from build123d import *

# Parameters (mm, degrees)
SKETCH_1_R          = 14.975
EXTRUDE_1_DEPTH     = 7
SKETCH_2_R          = 2.1
CUT_EXTRUDE_1_DEPTH = 10
SKETCH_3_R          = 1.65
CUT_EXTRUDE_2_DEPTH = 10
SKETCH_5_R          = 3.65
CUT_EXTRUDE_3_DEPTH = 4


with BuildPart() as part:
    # 草图1 → 凸台-拉伸1 (new body)
    with BuildSketch(Plane(origin=(0, 0, 0), x_dir=(1, 0, 0), z_dir=(0, 1, 0))):
        with Locations(Location((0, 0, 0), (0, 0, 270))):
            Circle(SKETCH_1_R)
    extrude(amount=EXTRUDE_1_DEPTH)

    # 草图2 → 切除-拉伸1 (cut)
    with BuildSketch(Plane(origin=(0, 7, 0), x_dir=(1, 0, 0), z_dir=(0, 1, 0))):
        with Locations(Location((-5, 0, 0), (0, 0, 270))):
            Circle(SKETCH_2_R)
        with Locations(Location((2.5, 4.330127019, 0), (0, 0, 270))):
            Circle(SKETCH_2_R)
        with Locations(Location((2.5, -4.330127019, 0), (0, 0, 270))):
            Circle(SKETCH_2_R)
    extrude(amount=-CUT_EXTRUDE_1_DEPTH, mode=Mode.SUBTRACT)

    # 草图3 → 切除-拉伸2 (cut)
    with BuildSketch(Plane(origin=(0, 7, 0), x_dir=(1, 0, 0), z_dir=(0, 1, 0))):
        with Locations(Location((0, 11, 0), (0, 0, 270))):
            Circle(SKETCH_3_R)
        with Locations(Location((9.526279442, 5.5, 0), (0, 0, 270))):
            Circle(SKETCH_3_R)
        with Locations(Location((9.526279442, -5.5, 0), (0, 0, 270))):
            Circle(SKETCH_3_R)
        with Locations(Location((0, -11, 0), (0, 0, 270))):
            Circle(SKETCH_3_R)
        with Locations(Location((-9.526279442, -5.5, 0), (0, 0, 270))):
            Circle(SKETCH_3_R)
        with Locations(Location((-9.526279442, 5.5, 0), (0, 0, 270))):
            Circle(SKETCH_3_R)
    extrude(amount=-CUT_EXTRUDE_2_DEPTH, mode=Mode.SUBTRACT)

    # 草图5 → 切除-拉伸3 (cut)
    with BuildSketch(Plane(origin=(0, 7, 0), x_dir=(1, 0, 0), z_dir=(0, 1, 0))):
        with Locations(Location((-5, 0, 0), (0, 0, 270))):
            Circle(SKETCH_5_R)
        with Locations(Location((2.5, 4.330127019, 0), (0, 0, 270))):
            Circle(SKETCH_5_R)
        with Locations(Location((2.5, -4.330127019, 0), (0, 0, 270))):
            Circle(SKETCH_5_R)
    extrude(amount=-CUT_EXTRUDE_3_DEPTH, mode=Mode.SUBTRACT)


solid = part.part
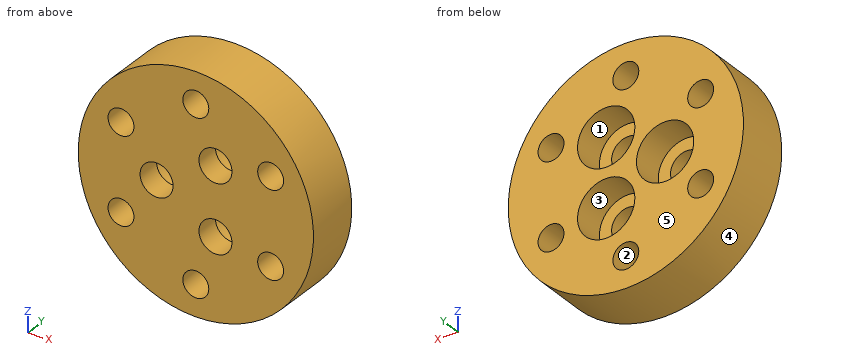
Verification items for the finished model (mm, model axes). Face numbers are marked on the shaded views. A direction names the side the tool comes from. Give positions to 0.01 mm unless a question says otherwise; leave off trailing zeros. Loops run counter-clockwise (first coordinate to the right, second up) from the corner with the lowest first, then second, coordinate; pieces in that order, holes last.
1) Thickness scan on line 1 along X through (y, z) = (2.25, 5.5); line 2 along Z through (x, y) = (4, 1.5); line 3 along X through (y, z) = (4.75, -6.5). Record the ranges inside material, lowest first.
2) Depth check by flat-ended pin: pin 1 Ø1.5 at (y, z) = (4.5, 7) entering from +X; pin 2 Ø2 at (x, z) = (4.5, 4.5) entering from +Y; pin 3 Ø2 at (x, y) = (-7.5, 3.5) entering from +Z. Enter the tip coordinate at first touch or a pass-through.
3) Sectioned sample at A-A, the plane z = 0. Enter the section's corners in (x, y) (3 decimals).
4) Sectioned sample at B-B, the plane z = -4.5. Enter the section's corners in (x, y), then the cut area to 3 significant figures.
5) Sectioned sample at C-C, the plane x = 2.5. Enter the section's corners in (y, z).
6) Draft check along Z on the marked faces 3, 4 and 5. Enter one of: pulls with the +Z half, pulls with the -Z half, needs draft (parallel to the pull), parting line crosses it, or undercut.
7) Set-up check for the marked faces 1 and 2: record each of +Z, -Z, +X, -X, +Y, -Y from which the full face is reachable in a straight line by a thin tool's end or side.
8) Sectioned sample at D-D, the plane y = 5.5. Count the separate pieces of the cut face and the enclosed holes in it, then the cut area to 3 significant figures.
Answers:
1. line 1: x = -13.93 to -11.18, -7.88 to 0.76, 4.24 to 7.88, 11.18 to 13.93
1. line 2: z = -14.43 to -5.8, -2.86 to 2.86, 5.8 to 14.43
1. line 3: x = -13.49 to -10.84, -8.21 to -0.43, 5.43 to 8.21, 10.84 to 13.49
2. pin 1: stops at x = 13.61
2. pin 2: stops at y = 3
2. pin 3: stops at z = 13.49
3. outline: (-14.975, 0) - (-7.1, 0) - (-7.1, 3) - (-8.65, 3) - (-8.65, 7) - (-14.975, 7) - close; (-2.9, 0) - (14.975, 0) - (14.975, 7) - (-1.35, 7) - (-1.35, 3) - (-2.9, 3) - close
4. outline: (-14.28, 0) - (-10.84, 0) - (-10.84, 7) - (-14.28, 7) - close; (-8.21, 0) - (0.41, 0) - (0.41, 3) - (-1.15, 3) - (-1.15, 7) - (-8.21, 7) - close; (4.59, 0) - (8.21, 0) - (8.21, 7) - (6.15, 7) - (6.15, 3) - (4.59, 3) - close; (10.84, 0) - (14.28, 0) - (14.28, 7) - (10.84, 7) - close
4. area: 121 mm2
5. outline: (0, -14.76) - (7, -14.76) - (7, -7.98) - (3, -7.98) - (3, -6.43) - (0, -6.43) - close; (0, -2.23) - (3, -2.23) - (3, -0.68) - (7, -0.68) - (7, 0.68) - (3, 0.68) - (3, 2.23) - (0, 2.23) - close; (0, 6.43) - (3, 6.43) - (3, 7.98) - (7, 7.98) - (7, 14.76) - (0, 14.76) - close
6. face 3: undercut
6. face 4: parting line crosses it
6. face 5: needs draft
7. face 1: +Y
7. face 2: +Y, -Y
8. separate pieces: 1
8. enclosed holes: 9
8. area: 528 mm2
